from build123d import *

# Parameters (mm, degrees)
SKETCH_W            = 124
SKETCH_H            = 18.5
SKETCH_R            = 0.5
PAD_DEPTH           = 6
HOLE_D              = 0.7
HOLE_DEPTH          = 25
HOLE_CBORE_D        = 1.6
HOLE_CBORE_DEPTH    = 2.1
CHAMFER_SIZE        = 0.2
SKETCH002_W         = 12
SKETCH002_H         = 18.5
SKETCH002_W_2       = 36
SKETCH002_H_2       = 3
PAD001_DEPTH        = 4
CHAMFER001_SIZE     = 0.4
SKETCH003_R         = 1.1
POCKET_DEPTH        = 10.001
CHAMFER002_SIZE     = 0.7
SKETCH004_W         = 8
SKETCH004_H         = 8.5
POCKET001_DEPTH     = 8
HOLE003_D           = 2
HOLE003_CBORE_D     = 4.1
HOLE003_CBORE_DEPTH = 2.1
FILLET_R            = 4
POCKET002_DEPTH     = 2.1


with BuildPart() as part:
    # Sketch → Pad (new body)
    with BuildSketch(Plane(origin=(0, 0, 0), x_dir=(-1, 0, 0), z_dir=(0, 0, -1))):
        with Locations((0, -6.75)):
            Rectangle(SKETCH_W, SKETCH_H)
        with Locations((-33.67, -3.81)):
            Circle(SKETCH_R, mode=Mode.SUBTRACT)
        with Locations((-31.745, -3.81)):
            Circle(SKETCH_R, mode=Mode.SUBTRACT)
        with Locations((-21.595, -3.81)):
            Circle(SKETCH_R, mode=Mode.SUBTRACT)
        with Locations((-19.67, -3.81)):
            Circle(SKETCH_R, mode=Mode.SUBTRACT)
        with Locations((19.67, -3.81)):
            Circle(SKETCH_R, mode=Mode.SUBTRACT)
        with Locations((21.595, -3.81)):
            Circle(SKETCH_R, mode=Mode.SUBTRACT)
        with Locations((31.745, -3.81)):
            Circle(SKETCH_R, mode=Mode.SUBTRACT)
        with Locations((33.67, -3.81)):
            Circle(SKETCH_R, mode=Mode.SUBTRACT)
    extrude(amount=PAD_DEPTH)

    # Hole
    with Locations(Plane.XY):
        with Locations((-30.48, -6.25), (-27.94, -6.25), (-25.4, -6.25), (-22.86, -6.25), (22.86, -6.25), (25.4, -6.25), (27.94, -6.25), (30.48, -6.25)):
            CounterBoreHole(HOLE_D / 2, HOLE_CBORE_D / 2, HOLE_CBORE_DEPTH, depth=HOLE_DEPTH)

    # Chamfer
    chamfer_edges = [part.edges().sort_by_distance(p)[0] for p in [
        (30.13, -6.25, -2.1),
        (27.59, -6.25, -2.1),
        (25.05, -6.25, -2.1),
        (22.51, -6.25, -2.1),
        (-30.83, -6.25, -2.1),
        (-28.29, -6.25, -2.1),
        (-25.75, -6.25, -2.1),
        (-23.21, -6.25, -2.1),
    ]]
    chamfer(chamfer_edges, length=CHAMFER_SIZE)

    # Sketch002 (on Face25 of Chamfer) → Pad001 (join)
    with BuildSketch(Plane.XY):
        with Locations((-56, -6.75)):
            Rectangle(SKETCH002_W, SKETCH002_H)
        with Locations((56, -6.75)):
            Rectangle(SKETCH002_W, SKETCH002_H)
        with Locations((0, 1)):
            Rectangle(SKETCH002_W_2, SKETCH002_H_2)
        Polygon((-46, -16), (-46, -8), (-43, -8), (-43, -13), (-36, -13), (-36, -16), align=None)
        Polygon((46, -16), (46, -8), (43, -8), (43, -13), (36, -13), (36, -16), align=None)
    extrude(amount=PAD001_DEPTH)

    # Chamfer001
    chamfer001_edges = [part.edges().sort_by_distance(p)[0] for p in [
        (34.17, -3.81, -6),
        (32.245, -3.81, -6),
        (22.095, -3.81, -6),
        (20.17, -3.81, -6),
        (-19.17, -3.81, -6),
        (-21.095, -3.81, -6),
        (-31.245, -3.81, -6),
        (-33.17, -3.81, -6),
    ]]
    chamfer(chamfer001_edges, length=CHAMFER001_SIZE)

    # Sketch003 (on Face23 of Chamfer001) → Pocket (cut, through all)
    with BuildSketch(Plane.XY.offset(4)):
        with Locations((-33.17, -1)):
            Circle(SKETCH003_R)
        with Locations((-20.17, -1)):
            Circle(SKETCH003_R)
        with Locations((-33.17, -6.75)):
            Circle(SKETCH003_R)
        with Locations((-20.17, -6.75)):
            Circle(SKETCH003_R)
        with Locations((-20.17, -12.5)):
            Circle(SKETCH003_R)
        with Locations((-33.17, -12.5)):
            Circle(SKETCH003_R)
        with Locations((20.17, -1)):
            Circle(SKETCH003_R)
        with Locations((33.17, -1)):
            Circle(SKETCH003_R)
        with Locations((20.17, -6.75)):
            Circle(SKETCH003_R)
        with Locations((33.17, -6.75)):
            Circle(SKETCH003_R)
        with Locations((33.17, -12.5)):
            Circle(SKETCH003_R)
        with Locations((20.17, -12.5)):
            Circle(SKETCH003_R)
    extrude(amount=-POCKET_DEPTH, mode=Mode.SUBTRACT)

    # Chamfer002
    chamfer002_edges = [part.edges().sort_by_distance(p)[0] for p in [
        (19.07, -6.75, -6),
        (19.07, -1, -6),
        (19.07, -12.5, -6),
        (32.07, -12.5, -6),
        (32.07, -6.75, -6),
        (32.07, -1, -6),
        (-34.27, -1, -6),
        (-34.27, -6.75, -6),
        (-34.27, -12.5, -6),
        (-21.27, -12.5, -6),
        (-21.27, -6.75, -6),
        (-21.27, -1, -6),
    ]]
    chamfer(chamfer002_edges, length=CHAMFER002_SIZE)

    # Sketch004 (on Face35 of Chamfer002) → Pocket001 (cut)
    with BuildSketch(Plane.XY.offset(4)):
        with Locations((-58, -6.75)):
            Rectangle(SKETCH004_W, SKETCH004_H)
        with Locations((58, -6.75)):
            Rectangle(SKETCH004_W, SKETCH004_H)
    extrude(amount=-POCKET001_DEPTH, mode=Mode.SUBTRACT)

    # Hole003 (through all)
    with Locations(Plane.XZ.offset(16)):
        with Locations((-58, 0), (58, 0)):
            CounterBoreHole(HOLE003_D / 2, HOLE003_CBORE_D / 2, HOLE003_CBORE_DEPTH)

    # Fillet
    fillet_edges = [part.edges().sort_by_distance(p)[0] for p in [
        (-62, 0, 4),
        (-62, -13.5, 4),
        (62, 0, 4),
        (62, -13.5, 4),
        (54, -6.75, -4),
        (-54, -6.75, -4),
    ]]
    fillet(fillet_edges, radius=FILLET_R)

    # Sketch015 (on Face1 of Fillet) → Pocket002 (cut)
    with BuildSketch(Plane(origin=(0, 2.5, 0), x_dir=(-1, 0, 0), z_dir=(0, 1, 0))):
        Polygon((-56.845299, 2), (-59.154701, 2), (-60.309401, 0), (-59.154701, -2), (-56.845299, -2), (-55.690599, 0), align=None)
        Polygon((55.690599, 0), (56.845299, -2), (59.154701, -2), (60.309401, 0), (59.154701, 2), (56.845299, 2), align=None)
    extrude(amount=-POCKET002_DEPTH, mode=Mode.SUBTRACT)


solid = part.part
Part model, mm, in its own coordinate system. A direction names the side the tool comes from. Give positions to 0.01 mm unless a question says otherwise; leave off trailing zeros. Put each result on its own line as item: value. Start each with the question number.
1) Probe probe 1 along X at (y, z) = (-10.75, 0.75); probe 2 along Y at (x, z) = (30.48, -0.65); probe 3 along Y at (x, z) = (-25.4, -4.4). List the from-to ranges inside material, lowest first.
2) Pull direction Y, two halves, no side cores. Call faces 4 (the cylindrical face through (20.678, -13.476, -2.613)), 5 (the flat face through (-62, -6.9, -4.4)), 6 (the flat face through (-57, 0.4, 1)): +Y half, -Y half, draft (parallel to the pull), parting line (faces both ways), or undercut.
3) 3-axis set-ups, long thin cutter, end or side, ignore diameter. For faces 1 (the flat face through (-56.26, 1.46, -0.99)), 2 (the flat face through (60, -7, -4)), 3 (the flat face through (-46, -12, 2)): which of +Z, -Z, +X, -X, +Y, -Y reach the whole face in a straight line?
4) Flat gauge pins, fed straight in: pin 1 (0.5 mm diameter, centred on x = 28, y = -6.5, fed in from +Z); pin 2 (1.2 mm diameter, centred on x = 58, z = 0, fed in from +Y); pin 3 (1.2 mm diameter, centred on y = -11.5, z = 1.5, fed in from -X); pin 4 (4.5 mm diameter, centred on y = -8, z = 1.5, fed in from +X). Where does each tip first touch, or does it go through?
Numbers:
1. probe 1: -54 to -50, -46 to -43, 43 to 46, 50 to 54
1. probe 2: -16 to -7.05, -5.45 to 2.5
1. probe 3: -16 to -6.6, -5.9 to 2.5
2. face 4: undercut
2. face 5: draft
2. face 6: +Y half
3. face 1: +Y
3. face 2: +Z, +X
3. face 3: +Z, +Y, -Y
4. pin 1: z = -2.14
4. pin 2: through
4. pin 3: x = -61.9
4. pin 4: x = 54.07
